Input: part model. Units: mm. Frame: model coordinates. A direction names the side the tool comes from. Round coordinates to 2 decimals unless told otherwise and drop trailing zeros. Loops run counter-clockwise (first coordinate to the right, second up) from the corner with the lowest first, then second, coordinate; pieces in that order, holes last. Notation, with made-up numbers: (82, 64.5) - (130, 64.5) arc R14 ccw to (130, 91.5) - close; hole circle Ø11 at (-6, -37.75). An arc over 180 degrees is marked (long way). Use CSV: the item, a comma, the result in double quotes. Start each with the question number.
1. Material intervals for probe 1 along X at (y, z) = (-3, 0); probe 2 along Y at (x, z) = (123, 12.5); probe 3 along X at (y, z) = (-2.5, 0), sorted ascending. Write a range as from..to.
2. Access query for faces 5 (the cylindrical face through (215.97, -3.13, -2.02)), 6 (the flat face through (6.35, -35, -50)). Directions: +Z, -Z, +X, -X, +Y, -Y. A direction counts if a zero-diameter tool reaches every point of the face in a straight line with its end or side. Return the directions, or none.
3. Pin query (flat end, axial travel): P1, Ø4, axis at y = -50, z = -38.5, coming from the +X side; P2, Ø11, axis at x = 139.7, z = 0, coming from the +Y side; P3, Ø20, axis at y = -33.34, z = 0, coming from the -X side. Return the tip coordinate at first contact, or that it passes through.
4. Cut plane B-B (z = 0). Return loops of the section in (x, y), and give its area (3 significant figures).
5. Pull-direction query (Z, two-part tool) for faces 1 (the cylindrical face through (3.13, -41.89, 1.9)), 2 (the flat face through (98, 0, -33)), 3 (the flat face through (6, -22, -127)), 4 (the flat face through (89, -5, 25.4)); classes: +Z half, -Z half, draft (parallel to the pull), parting line (faces both ways), or undercut.
6. Cut plane A-A (x = 139.7). Return loops of the section in (y, z), and give its area (3 significant figures).
7. Cut plane D-D (z = -80). Return loops of the section in (x, y), and give its area (3 significant figures).
8. Cut plane C-C (y = -36). Return loops of the section in (x, z).
```python
from build123d import *

# Parameters (mm, degrees)
EXTRUDE1_DEPTH         = 127
SKETCH2_R              = 6.731
CUT_CHAMFER_DEPTH      = 508
CUT_CHAMFER_DEPTH_BACK = 58.15
SKETCH3_R              = 8.763
CUT_HOLES_DEPTH        = 229.6
CUT_LH_DEPTH           = 1
CUT_LH_DEPTH_BACK      = 58.15


with BuildPart() as part:
    # Sketch1 → Extrude1 (new body, symmetric)
    with BuildSketch(Plane.XY):
        with BuildLine():
            Line((228.6, 0), (12.7, 0))
            ThreePointArc((12.7, 0), (3.719743879, -3.719743879), (0, -12.7))
            Line((0, -12.7), (0, -57.15))
            Line((0, -57.15), (6.35, -57.15))
            Line((6.35, -57.15), (6.35, -12.7))
            ThreePointArc((6.35, -12.7), (8.209871939, -8.209871939), (12.7, -6.35))
            Line((12.7, -6.35), (228.6, -6.35))
            Line((228.6, -6.35), (228.6, 0))
        make_face()
    extrude(amount=EXTRUDE1_DEPTH, both=True)

    # Sketch2 → Cut-Chamfer (cut, two sides)
    with BuildSketch(Plane(origin=(0, 0, 0), x_dir=(1, 0, 0), z_dir=(0, 1, 0))) as cut_chamfer_sk:
        with Locations((209.55, 0)):
            Circle(SKETCH2_R)
        with Locations((139.7, 0)):
            Circle(SKETCH2_R)
        Polygon((25.4, 127), (228.6, 25.4), (228.6, 127), align=None)
        Polygon((25.4, -127), (228.6, -25.4), (228.6, -127), align=None)
    extrude(amount=CUT_CHAMFER_DEPTH, mode=Mode.SUBTRACT)
    extrude(cut_chamfer_sk.sketch, amount=-CUT_CHAMFER_DEPTH_BACK, mode=Mode.SUBTRACT)

    # Sketch3 → Cut-Holes (cut, through all)
    with BuildSketch(Plane(origin=(0, 0, 0), x_dir=(0, 0, -1), z_dir=(1, 0, 0))):
        with Locations((0, -33.3375)):
            Circle(SKETCH3_R)
        with Locations((101.6, -33.3375)):
            Circle(SKETCH3_R)
        with Locations((0, -153.9875)):
            Circle(SKETCH3_R)
        with Locations((101.6, -153.9875)):
            Circle(SKETCH3_R)
        with Locations((-101.6, -33.3375)):
            Circle(SKETCH3_R)
        with Locations((-101.6, -153.9875)):
            Circle(SKETCH3_R)
    extrude(amount=CUT_HOLES_DEPTH, mode=Mode.SUBTRACT)

    # Sketch5 → Cut-LH (cut, two sides)
    with BuildSketch(Plane(origin=(0, 0, 0), x_dir=(1, 0, 0), z_dir=(0, 1, 0))) as cut_lh_sk:
        Polygon((788.086014381, -25.4), (228.6, -25.4), (0, -25.4), (-559.486014381, -25.4), (-559.486014381, -1144.372028761), (788.086014381, -1144.372028761), align=None)
    extrude(amount=CUT_LH_DEPTH, mode=Mode.SUBTRACT)
    extrude(cut_lh_sk.sketch, amount=-CUT_LH_DEPTH_BACK, mode=Mode.SUBTRACT)


solid = part.part
```
Established:
1,probe 1,"x = 4.5..132.97, 146.43..202.82, 216.28..228.6"
1,probe 2,"y = -6.35..0"
1,probe 3,"x = 5.13..132.97, 146.43..202.82, 216.28..228.6"
2,face 5,"+Y, -Y"
2,face 6,"+Z, -Z, +X, -Y"
3,P1,"stops at x = 6.35"
3,P2,"passes through"
3,P3,"stops at x = 0"
4,outline,"(0, -57.15) - (6.35, -57.15) - (6.35, -42.1) - (0, -42.1) - close; (0, -24.57) - (6.35, -24.57) - (6.35, -12.7) arc R6.35 cw to (12.7, -6.35) - (132.97, -6.35) - (132.97, 0) - (12.7, 0) arc R12.7 ccw to (0, -12.7) - close; (146.43, -6.35) - (202.82, -6.35) - (202.82, 0) - (146.43, 0) - close; (216.28, -6.35) - (228.6, -6.35) - (228.6, 0) - (216.28, 0) - close"
4,area,"1,470 mm2"
5,face 1,"undercut"
5,face 2,"draft"
5,face 3,"-Z half"
5,face 4,"+Z half"
6,outline,"(-6.35, -69.85) - (0, -69.85) - (0, -6.73) - (-6.35, -6.73) - close; (-6.35, 6.73) - (0, 6.73) - (0, 25.4) - (-6.35, 25.4) - close"
6,area,"519 mm2"
7,outline,"(0, -57.15) - (6.35, -57.15) - (6.35, -12.7) arc R6.35 cw to (12.7, -6.35) - (119.4, -6.35) - (119.4, 0) - (12.7, 0) arc R12.7 ccw to (0, -12.7) - close"
7,area,"1,050 mm2"
8,outline,"(0, -127) - (6.35, -127) - (6.35, -109.95) - (0, -109.95) - close; (0, -93.25) - (6.35, -93.25) - (6.35, -8.35) - (0, -8.35) - close; (0, 8.35) - (6.35, 8.35) - (6.35, 25.4) - (0, 25.4) - close"
